Here's how the part is built. I have some questions about the finished solid (model axes, mm). A direction names the side the tool comes from. Give positions to 0.01 mm unless a question says otherwise; leave off trailing zeros. Loops run counter-clockwise (first coordinate to the right, second up) from the corner with the lowest first, then second, coordinate; pieces in that order, holes last.
Q1. I need wall thicknesses on probe 1 along Z at (x, y) = (0, -4); probe 2 along Z at (x, y) = (-20.5, 24.5); probe 3 along X at (y, z) = (-2, 1). Which ranges of each line are inside material? Lowest first, please.
Q2. Suppose I cut it at C-C (y = 24). List the corners of the cut face in (x, z) for me.
Q3. For faces 4 (the face through (-1.73, -7.81, 9.96)), 5 (the face through (-3, -1, 15)), which set-ups out of +Z, -Z, +X, -X, +Y, -Y let a thin tool reach every point of the face, with its end or its side?
Q4. Thinking about a two-plate mould opening in X: for faces 1 (the face through (-0.7, -10.4, 5)), 2 (the face through (2.77, -1.15, 5.14)), 3 (the face through (47.69, 15.02, 0.07)), which applies, pulls with the +X half, pulls with the -X half, needs draft (parallel to the pull), parting line crosses it, or undercut?
Q5. I'm going to push flat-ended pins straight in: P1, Ø10, axis at y = -33, z = 4.5, coming from the -X side; P2, Ø12, axis at y = -25.5, z = 0.5, coming from the -X side; P3, Ø5, axis at y = 36, z = -1.5, coming from the +X side. Where does each tip first touch, or does it pass through?
Q6. Suppose I cut it at A-A (y = 0). List the corners of the cut face in (x, z) for me, and give its area (3 significant figures).
Q7. Suppose I cut it at B-B (x = 33). List the corners of the cut face in (y, z) for me, and give its area (3 significant figures).
```python
from build123d import *

# Parameters (mm, degrees)
SKETCH1_R               = 50
BOSS_EXTRUDE1_DEPTH     = 5
SKETCH2_R               = 8
BOSS_EXTRUDE2_DEPTH     = 10
SKETCH3_R               = 3
CUT_EXTRUDE1_DEPTH      = 74.484692283
FILLET1_R               = 2
CUT_EXTRUDE2_DEPTH      = 73.284161474
CUT_EXTRUDE2_DEPTH_BACK = 73.284161474
SKETCH4_R               = 1


with BuildPart() as part:
    # Sketch1 → Boss-Extrude1 (new, symmetric)
    with BuildSketch(Plane.XY):
        Circle(SKETCH1_R)
    extrude(amount=BOSS_EXTRUDE1_DEPTH, both=True)

    # Sketch2 → Boss-Extrude2 (add)
    with BuildSketch(Plane.XY.offset(5)):
        Circle(SKETCH2_R)
    extrude(amount=BOSS_EXTRUDE2_DEPTH)

    # Sketch3 → Cut-Extrude1 (cut, through all)
    with BuildSketch(Plane.XY.offset(15)):
        Circle(SKETCH3_R)
    extrude(amount=-CUT_EXTRUDE1_DEPTH, mode=Mode.SUBTRACT)

    # Fillet1
    fillet1_edges = [part.edges().sort_by_distance(p)[0] for p in [
        (-8, 0, 5),
        (-8, 0, 15),
    ]]
    fillet(fillet1_edges, radius=FILLET1_R)

    # Sketch4 → Cut-Extrude2 (cut, two sides: drawn at the far end of the back side and taken through both)
    with BuildSketch(Plane(origin=(0, 0, 0), x_dir=(1, 0, 0), z_dir=(0, 1, 0)).offset(-CUT_EXTRUDE2_DEPTH_BACK)):
        with Locations(Location((0, -10, 0), (0, 0, 270))):
            Circle(SKETCH4_R)
    extrude(amount=CUT_EXTRUDE2_DEPTH + CUT_EXTRUDE2_DEPTH_BACK, mode=Mode.SUBTRACT)


solid = part.part
```
Solutions:
1. probe 1: z = -5 to 9, 11 to 15
1. probe 2: z = -5 to 5
1. probe 3: x = -49.96 to -2.24, 2.24 to 49.96
2. outline: (-43.86, -5) - (43.86, -5) - (43.86, 5) - (-43.86, 5) - close
3. face 4: +Z
3. face 5: +Z, +X, -X, +Y, -Y
4. face 1: needs draft
4. face 2: undercut
4. face 3: parting line crosses it
5. P1: stops at x = -41.42
5. P2: stops at x = -46.04
5. P3: stops at x = 37.12
6. outline: (-50, -5) - (-3, -5) - (-3, 15) - (-6, 15) arc R2 ccw to (-8, 13) - (-8, 7) arc R2 cw to (-10, 5) - (-50, 5) - close; (3, -5) - (50, -5) - (50, 5) - (10, 5) arc R2 cw to (8, 7) - (8, 13) arc R2 ccw to (6, 15) - (3, 15) - close
6. area: 1,040 mm2
7. outline: (-37.56, -5) - (37.56, -5) - (37.56, 5) - (-37.56, 5) - close
7. area: 751 mm2
